Geometry check sheet. Reference: the model listing, model coordinates, mm. Face numbers are marked on the shaded views. Give positions to 0.01 mm unless a question says otherwise; leave off trailing zeros. Write each loop counter-clockwise with the first axis right and the second up, starting at its lowest first coordinate (ties: lowest second). Pieces come first, ordered by that corner, then holes. Notation, with made-up numbers: (9.5, -30.5) -> (19.5, -30.5) arc R11 cw to (19.5, -24.5) -> close; hole circle Ø8 at (10.5, 11.25). An arc over 180 degrees is marked (long way). One line per item, written item: value.
from build123d import *

# Parameters (mm, degrees)
SKETCH_1_W                   = 19
SKETCH_1_H                   = 8
EXTRUDE_1_DEPTH              = 1.75
CUT_EXTRUDE_1_REACH          = 14.542
SKETCH_2_W                   = 7.5
SKETCH_2_H                   = 1.8
HOLE_WIZARD_M3_1_D           = 3.2
HOLE_WIZARD_M3_1_CSINK_D     = 6
HOLE_WIZARD_M3_1_CSINK_ANGLE = 90
FILLET_2_R                   = 4
FILLET_3_R                   = 0.5
CHAMFER_1_SIZE               = 0.3


with BuildPart() as part:
    # 草图1 → 凸台-拉伸1 (new, symmetric)
    with BuildSketch(Plane(origin=(0, 0, 0), x_dir=(1, 0, 0), z_dir=(0, 1, 0))):
        Rectangle(SKETCH_1_W, SKETCH_1_H)
    extrude(amount=EXTRUDE_1_DEPTH, both=True)

    # 草图2 → 切除-拉伸1 (cut, up to next)
    with BuildSketch(Plane.XY.offset(4), mode=Mode.PRIVATE) as cut_extrude_1_sk1:
        with Locations((0, -0.85)):
            Rectangle(SKETCH_2_W, SKETCH_2_H)
    cut_extrude_1_tool1 = extrude(cut_extrude_1_sk1.sketch, amount=-CUT_EXTRUDE_1_REACH, mode=Mode.PRIVATE) & part.part
    add(cut_extrude_1_tool1.solids().sort_by_distance((0, -0.85, 4))[0], mode=Mode.SUBTRACT)

    # M3 十字槽半沉头木螺钉的锥形沉头孔1 (through all)
    with Locations(Plane(origin=(0, 1.75, 0), x_dir=(1, 0, 0), z_dir=(0, 1, 0))):
        with Locations((6, 0), (-6, 0)):
            CounterSinkHole(HOLE_WIZARD_M3_1_D / 2, HOLE_WIZARD_M3_1_CSINK_D / 2, counter_sink_angle=HOLE_WIZARD_M3_1_CSINK_ANGLE)

    # 圆角2
    fillet_2_edges = [part.edges().sort_by_distance(p)[0] for p in [
        (9.5, 0, 4),
        (-9.5, 0, -4),
        (9.5, 0, -4),
        (-9.5, 0, 4),
    ]]
    fillet(fillet_2_edges, radius=FILLET_2_R - 0.0001)  # a hair under: the kernel refuses the full size

    # 圆角3
    fillet_3_edges = [part.edges().sort_by_distance(p)[0] for p in [
        (3.75, 0.05, 0),
        (3.75, -1.75, 0),
        (-3.75, -1.75, 0),
        (-3.75, 0.05, 0),
    ]]
    fillet(fillet_3_edges, radius=FILLET_3_R)

    # 倒角1
    chamfer_1_edges = [part.edges().sort_by_distance(p)[0] for p in [
        (0, 1.75, 4),
        (0, 1.75, -4),
        (-8.328456414, 1.75, 2.828456414),
        (-8.328456414, 1.75, -2.828456414),
        (8.328456414, 1.75, -2.828456414),
        (8.328456414, 1.75, 2.828456414),
    ]]
    chamfer(chamfer_1_edges, length=CHAMFER_1_SIZE)


solid = part.part
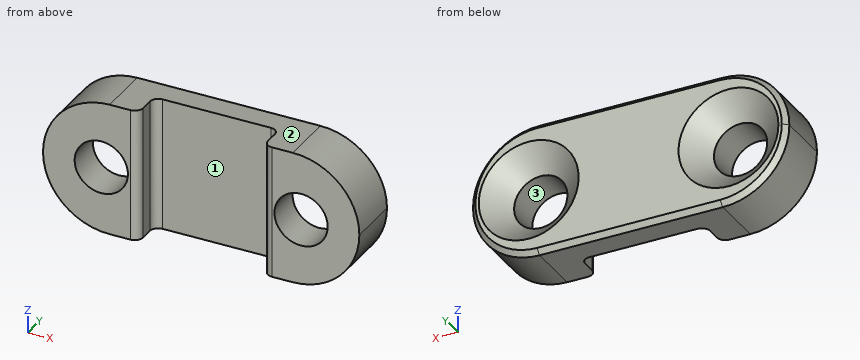
1) Sectioned sample at C-C on x = -2. Record the cut outline in (y, z), plus the area to 3 significant figures.
Verdict:
outline: (0.05, -4) -> (1.45, -4) -> (1.75, -3.7) -> (1.75, 3.7) -> (1.45, 4) -> (0.05, 4) -> close
area: 13.5 mm^2
2) Depth check by flat-ended pin: pin 1 Ø0.9 at (y, z) = (-0.5, 1.5) entering from -X; pin 2 Ø4 at (x, z) = (-5.5, -0.5) entering from +Y. Enter the tip coordinate at first touch or a pass-through.
Verdict:
pin 1: x = -9.36
pin 2: y = 1.46
3) Mould release check, pull along Z, two halves, no side actions. Record for the marked faces 1, 2 and 3: released by +Z, released by -Z, zero draft, split by the parting line, or undercut.
Verdict:
face 1: zero draft
face 2: released by +Z
face 3: undercut
4) Sectioned sample at A-A on y = 1. Give the number of separate pieces and of enclosed holes in the cut face, plus the area to 3 significant figures.
Verdict:
separate pieces: 1
enclosed holes: 2
area: 106 mm^2
5) Scan lines: probe 1 along X at (y, z) = (-0.4, -1); probe 2 along X at (y, z) = (0.6, 1); probe 3 along X at (y, z) = (1, -0.25). Record each from-to range of solid material in increasing order.
Verdict:
probe 1: -9.37 to -7.25, -4.75 to -3.75, 3.75 to 4.75, 7.25 to 9.37
probe 2: -9.37 to -7.56, -4.44 to 4.44, 7.56 to 9.37
probe 3: -9.49 to -8.24, -3.76 to 3.76, 8.24 to 9.49
